Geometry check sheet. Reference: the model listing, model coordinates, mm. Round coordinates to 2 decimals unless told otherwise and drop trailing zeros. Order: outer loops, then holes, each group sorted by start corner. A loop starts at its lowest first (then second) coordinate and runs counter-clockwise, first axis right, second up.
(1) Cross-section at B-B on y = -67. Enter the section's corners in (x, z), and give its area (3 significant figures).
(2) Cross-section at A-A on z = 4.5. Enter the section's corners in (x, y) (1 decimal).
(3) Gauge pin test, flat end, axial feed: P1, Ø15.5, axis at x = -37.63, y = -70.59, coming from the -Z side. Record the tip position at first contact, or that the pin passes through.
(4) Thickness scan on L1, parallel to Y at x = -37.5, z = 6; L2, parallel to Y at x = -42, z = 3.25; L3, parallel to X at y = -135.5, z = 2.75. Record the ranges inside material, lowest first.
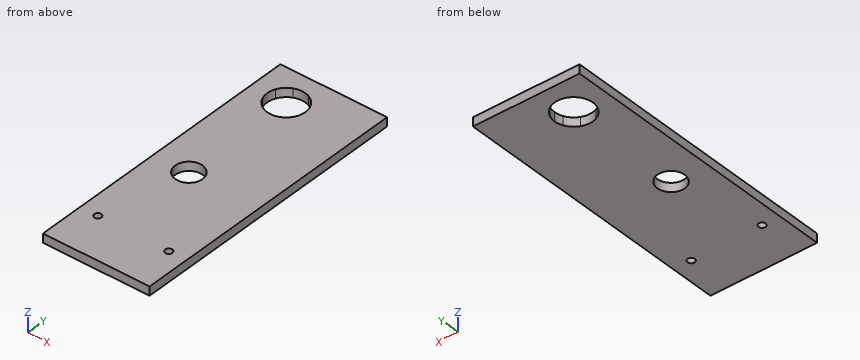
from build123d import *

# Parameters (mm, degrees)
SKETCH1_W           = 76.2
SKETCH1_H           = 203.2
BOSS_EXTRUDE1_DEPTH = 6.35
SKETCH2_R           = 9.779
SKETCH2_R_2         = 2.5527
CUT_EXTRUDE1_DEPTH  = 6.35
CUT_EXTRUDE3_DEPTH  = 6.35


with BuildPart() as part:
    # Sketch1 → Boss-Extrude1 (new body)
    with BuildSketch(Plane.XY):
        with Locations((-24.805306972, -63.605723205)):
            Rectangle(SKETCH1_W, SKETCH1_H)
    extrude(amount=BOSS_EXTRUDE1_DEPTH)

    # Sketch2 → Cut-Extrude1 (cut)
    with BuildSketch(Plane.XY.offset(6.35)):
        with Locations((-37.632306972, -70.590723205)):
            Circle(SKETCH2_R)
        with Locations((-50.205306972, -133.455723205)):
            Circle(SKETCH2_R_2)
        with Locations((0.594693028, -133.455723205)):
            Circle(SKETCH2_R_2)
    extrude(amount=-CUT_EXTRUDE1_DEPTH, mode=Mode.SUBTRACT)

    # Sketch7 → Cut-Extrude3 (cut)
    with BuildSketch(Plane.XY.offset(6.35)):
        with BuildLine():
            Line((-37.759306972, 25.294276795), (-37.759306972, 0.402276795))
            Line((-37.759306972, 0.402276795), (-32.147904273, 0.402276795))
            ThreePointArc((-32.147904273, 0.402276795), (-28.105531642, 3.194501465), (-25.313306972, 7.236874096))
            Line((-25.313306972, 7.236874096), (-25.313306972, 18.459679494))
            ThreePointArc((-25.313306972, 18.459679494), (-28.105531642, 22.502052125), (-32.147904273, 25.294276795))
            Line((-32.147904273, 25.294276795), (-37.759306972, 25.294276795))
        make_face()
        with BuildLine():
            Line((-25.313306972, 18.459679494), (-25.313306972, 7.236874096))
            ThreePointArc((-25.313306972, 7.236874096), (-24.411839586, 9.978456134), (-24.106806972, 12.848276795))
            ThreePointArc((-24.106806972, 12.848276795), (-24.411839586, 15.718097456), (-25.313306972, 18.459679494))
        make_face()
        with BuildLine():
            Line((-43.370709671, 25.294276795), (-37.759306972, 25.294276795))
            Line((-37.759306972, 25.294276795), (-32.147904273, 25.294276795))
            ThreePointArc((-32.147904273, 25.294276795), (-37.759306972, 26.500776795), (-43.370709671, 25.294276795))
        make_face()
        with BuildLine():
            Line((-32.147904273, 0.402276795), (-37.759306972, 0.402276795))
            Line((-37.759306972, 0.402276795), (-43.370709671, 0.402276795))
            ThreePointArc((-43.370709671, 0.402276795), (-37.759306972, -0.804223205), (-32.147904273, 0.402276795))
        make_face()
        with BuildLine():
            Line((-43.370709671, 0.402276795), (-37.759306972, 0.402276795))
            Line((-37.759306972, 0.402276795), (-37.759306972, 25.294276795))
            Line((-37.759306972, 25.294276795), (-43.370709671, 25.294276795))
            ThreePointArc((-43.370709671, 25.294276795), (-47.413082302, 22.502052125), (-50.205306972, 18.459679494))
            Line((-50.205306972, 18.459679494), (-50.205306972, 7.236874096))
            ThreePointArc((-50.205306972, 7.236874096), (-47.413082302, 3.194501465), (-43.370709671, 0.402276795))
        make_face()
        with BuildLine():
            ThreePointArc((-50.205306972, 18.459679494), (-51.411806972, 12.848276795), (-50.205306972, 7.236874096))
            Line((-50.205306972, 7.236874096), (-50.205306972, 18.459679494))
        make_face()
    extrude(amount=-CUT_EXTRUDE3_DEPTH, mode=Mode.SUBTRACT)


solid = part.part
Found:
1. outline: (-62.91, 0) - (-46.73, 0) - (-46.73, 6.35) - (-62.91, 6.35) - close; (-28.54, 0) - (13.29, 0) - (13.29, 6.35) - (-28.54, 6.35) - close
1. area: 368 mm2
2. outline: (-62.9, -165.2) - (13.3, -165.2) - (13.3, 38) - (-62.9, 38) - close; hole circle Ø5.1 at (-50.2, -133.5); hole circle Ø27.3 at (-37.8, 12.8); hole circle Ø19.6 at (-37.6, -70.6); hole circle Ø5.1 at (0.6, -133.5)
3. P1: passes through
4. L1: y = -165.21 to -80.37, -60.81 to -0.8, 26.5 to 37.99
4. L2: y = -165.21 to -79.34, -61.84 to -0.13, 25.83 to 37.99
4. L3: x = -62.91 to -51.73, -48.68 to -0.93, 2.12 to 13.29
